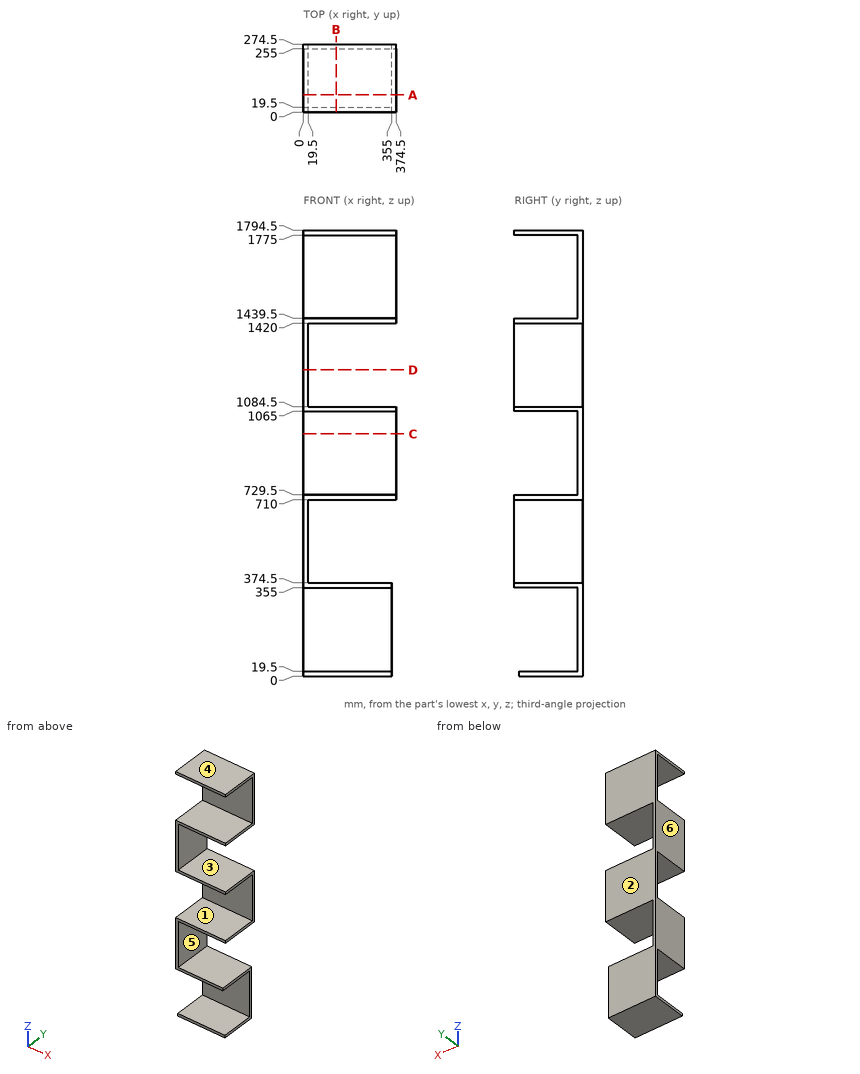
For this review, use the dimensioned drawing (mm, ordinates from the lowest corner) and the shaded views. A direction names the side the tool comes from. Give positions to 0.01 mm unless a question says otherwise; leave off trailing zeros. Order: outer loops, then holes, each group sorted by start corner. A loop starts at its lowest first (then second) coordinate and runs counter-clockwise, first axis right, second up. Notation, with made-up numbers: (66.25, -29) - (96.25, -29) arc R19 cw to (96.25, -23) - close; hole circle Ø11 at (31, 41). An arc over 180 degrees is marked (long way). Use a Markdown table: item, result. Add a question column.
(1) Mouldability with a two-part tool opening along Z and no side actions: class the marked faces 4, 5 and 6 as +Z half, -Z half, draft (parallel to the pull), parting line (faces both ways), or undercut.
(2) Wall thickness on probe 1 along Z at (x, y) = (140, 204.5); probe 2 along X at (y, z) = (249.5, 1418); probe 3 along X at (y, z) = (263.5, 124): over which ranges is each line inside the solid? List them lowest first. Write a range as [from, to].
(3) Add section C-C on z = 974.5. Give the boundary of the cut face in (x, y), then the cut area to 3 significant figures.
(4) Clearance check with flat-ended pins moving along their axes: P1, Ø4, axis at x = 123, z = 825.5, coming from the -Y side; P2, Ø1, axis at x = 300, y = 57, coming from the -Z side; P3, Ø10, axis at x = 167.5, z = 6.5, coming from the -Y side. State where each tip first meets the part, or that it passes through.
(5) Add section B-B on x = 132. Give the boundary of the cut face in (y, z).
(6) Add section D-D on z = 1232.5. Give the boundary of the cut face in (x, y).
(7) Machinability: for the marked faces 1, 2 and 3, which of the approach directions +Z, -Z, +X, -X, +Y, -Y give a long, thin tool a straight path to every point of the face, cutting with its end or side? Answer none if there is none.
(8) Add section A-A on y = 70. Give the boundary of the cut face in (x, z), then the cut area to 3 significant figures.
Report:
| question | item | result |
|---|---|---|
| 1 | face 4 | +Z half |
| 1 | face 5 | undercut |
| 1 | face 6 | draft |
| 2 | probe 1 | z = [0, 19.5], [355, 374.5], [710, 729.5], [1065, 1084.5], [1420, 1439.5], [1775, 1794.5] |
| 2 | probe 2 | x = [0, 19.5] |
| 2 | probe 3 | x = [0, 355] |
| 3 | outline | (0, 255) - (374.5, 255) - (374.5, 274.5) - (0, 274.5) - close |
| 3 | area | 7,300 mm² |
| 4 | P1 | stops at y = 255 |
| 4 | P2 | stops at z = 0 |
| 4 | P3 | stops at y = 19.5 |
| 5 | outline | (0, 355) - (255, 355) - (255, 19.5) - (19.5, 19.5) - (19.5, 0) - (274.5, 0) - (274.5, 374.5) - (0, 374.5) - close; (0, 710) - (274.5, 710) - (274.5, 1084.5) - (0, 1084.5) - (0, 1065) - (255, 1065) - (255, 729.5) - (0, 729.5) - close; (0, 1420) - (274.5, 1420) - (274.5, 1794.5) - (0, 1794.5) - (0, 1775) - (255, 1775) - (255, 1439.5) - (0, 1439.5) - close |
| 6 | outline | (0, 0) - (19.5, 0) - (19.5, 274.5) - (0, 274.5) - close |
| 7 | face 1 | +X, -X, -Y |
| 7 | face 2 | +Z, -Z, +X, -X, +Y |
| 7 | face 3 | +X, +Y, -Y |
| 8 | outline | (0, 0) - (355, 0) - (355, 19.5) - (0, 19.5) - close; (0, 355) - (355, 355) - (355, 374.5) - (19.5, 374.5) - (19.5, 710) - (374.5, 710) - (374.5, 729.5) - (0, 729.5) - close; (0, 1065) - (374.5, 1065) - (374.5, 1084.5) - (19.5, 1084.5) - (19.5, 1420) - (374.5, 1420) - (374.5, 1439.5) - (0, 1439.5) - close; (0, 1775) - (374.5, 1775) - (374.5, 1794.5) - (0, 1794.5) - close |
| 8 | area | 56,100 mm² |
